Work out the finished part from the listing and answer in its coordinate system (mm). A direction names the side the tool comes from. Coordinates: 2 decimals unless noted, no trailing zeros. Write each loop counter-clockwise with the first axis right and the second up, starting at its lowest first coordinate (ties: lowest second). Pieces come first, ordered by that corner, then holes. Notation, with made-up numbers: (-19.5, 67) - (10.5, 67) arc R15 ccw to (10.5, 76) - close; hole circle Ø5 at (24.25, -29.75). An arc over 180 degrees is marked (long way). One line per item, written item: value.
Autodesk Inventor part; units mm, degrees
ref_plane "YZ Plane" through (0, 0, 0) normal (1, 0, 0) x (0, 1, 0)
ref_plane "XZ Plane" through (0, 0, 0) normal (0, 1, 0) x (-1, 0, 0)
ref_plane "XY Plane" through (0, 0, 0) normal (0, 0, 1) x (1, 0, 0)
sketch "Sketch2" plane through (0, 0, 0) normal (0, 1, 0) x (-1, 0, 0)
  line L0 (0, 0) -> (0, 50)
  line L1 (0, 50) -> (30, 50)
  line L2 (30, 50) -> (30, 0)
  line L3 (0, 0) -> (-50, 0)
  line L4 (0, 0) -> (50, 0) construction
  line L5 (-50, 0) -> (-50, -30)
  line L6 (-50, -30) -> (30, -30)
  line L7 (30, -30) -> (30, 0)
  dimension "d7" = 50
  dimension "d8" = 30
  dimension "d9" = 90
  dimension "d10" = 50
  dimension "d11" = 90
  dimension "d12" = 50
  dimension "d13" = 180
  dimension "d14" = 30
  dimension "d15" = 90
extrude "Extrusion1" add sketch "Sketch2" along normal blind 20
sketch "Sketch3" plane through (0, 0, 50) normal (1, 0, 0) x (0, 0, -1)
  line L0 (0, 5) -> (75, 5)
  line L1 (75, 5) -> (75, 15)
  line L2 (75, 15) -> (0, 15)
  line L3 (0, 15) -> (0, 5)
  point P0 (50, 0)
  dimension "d18" = 10
extrude "Extrusion2" cut sketch "Sketch3" against normal blind 25
sketch "Sketch4" plane through (0, 0, 0) normal (0, 0, 1) x (1, 0, 0)
  line L0 (0, 15) -> (-25, 15)
  line L1 (-25, 15) -> (75, 15)
  line L2 (75, 15) -> (75, 5)
  line L3 (75, 5) -> (-25, 5)
  line L4 (-25, 5) -> (-25, 15)
  point P0 (0, 0)
  dimension "d21" = 100
  dimension "d22" = 10
extrude "Extrusion3" cut sketch "Sketch4" against normal blind 25
properties part number "TSU_Corner_Clamp"
Item 1: Section C-C, the plane y = 2 is taken. Determine the outline of the cut face in (x, z), then the cut area to 3 significant figures.
Evaluation:
outline: (-30, -30) - (50, -30) - (50, 0) - (0, 0) - (0, 50) - (-30, 50) - close
area: 3,900 mm2
Item 2: Section B-B, the plane x = 36 is taken. Determine the outline of the cut face in (y, z).
Evaluation:
outline: (0, -30) - (20, -30) - (20, 0) - (15, 0) - (15, -25) - (5, -25) - (5, 0) - (0, 0) - close
Item 3: Section D-D, the plane y = 7 is taken. Determine the outline of the cut face in (x, z).
Evaluation:
outline: (-30, -30) - (50, -30) - (50, -25) - (-25, -25) - (-25, 50) - (-30, 50) - close
Item 4: Section A-A, the plane z = -21 is taken. Determine the outline of the cut face in (x, y).
Evaluation:
outline: (-30, 0) - (50, 0) - (50, 5) - (-25, 5) - (-25, 15) - (50, 15) - (50, 20) - (-30, 20) - close
Item 5: Which of the six approach directions +Z, -Z, +X, -X, +Y, -Y give full straight-line access (tool end or side, diameter ignored) to faces 1 (the face through (-7, 20, 2)), 2 (the face through (-4, 15, 4)), 3 (the face through (0, 2, 25))?
Evaluation:
face 1: +Z, -Z, +X, -X, +Y
face 2: +Z, +X
face 3: +Z, +X, +Y, -Y
Item 6: Given pin 1 (4 mm diameter, centred on x = 22, y = 18, fed in from +Z); pin 2 (11 mm diameter, centred on y = 10, z = 26, fed in from +X); pin 3 (1.5 mm diameter, centred on y = 9, z = -22, fed in from +X); pin 4 (22.5 mm diameter, centred on x = 27, z = 15.5, fed in from +Y), each flat-ended and moving along its own axis, determine where each tip first touches the part or whether it passes through.
Evaluation:
pin 1: stops at z = 0
pin 2: stops at x = 0
pin 3: stops at x = -25
pin 4: passes through
Item 7: Consider probe 1 along Y at (x, z) = (41, -16.5); probe 2 along X at (y, z) = (7.5, 11.5); probe 3 along X at (y, z) = (15.25, 44.5). Determine where each line is inside the solid, lowest interval first.
Evaluation:
probe 1: y = 0 to 5, 15 to 20
probe 2: x = -30 to -25
probe 3: x = -30 to 0
